Answer from the drawing. Dimensions are ordinates in mm from the lowest x, y and z of the part. Coordinates: 2 decimals unless noted, no trailing zeros. Loops run counter-clockwise (first coordinate to the right, second up) from the corner with the lowest first, then second, coordinate; pieces in that order, holes last. Notation, with made-up numbers: (69, 51.25) - (121, 51.25) arc R18 cw to (121, 65.25) - close; hole circle Ø1 at (73, 75.5). An arc over 180 degrees is marked (long way). Write each question's results on one line, items separated by ' | '. Start each with the question number.
1. A cutting plane is placed at A-A on x = 20. Determine the outline of the cut face in (y, z) (1 decimal), then the cut area to 3 significant figures.
2. A cutting plane is placed at D-D on x = 6. Determine the outline of the cut face in (y, z) (1 decimal), then the cut area to 3 significant figures.
3. This flat-tipped pin is pushed along its axis until it touches: P1, Ø1, axis at x = 23.5, y = 21, coming from the -Z side. Where does it stop, or does it pass through?
4. Determine the mould class of the marked faces 1, 2 and 3 for opening direction Z: released by +Z, released by -Z, zero draft, split by the parting line, or undercut.
5. Find the intervals of material crossed by line 1 along X through (y, z) = (19.75, 25.5); line 2 along Z through (x, y) = (33, 6.5) (1 decimal); line 3 along Z through (x, y) = (21, 18.5) (1 decimal), in increasing order. Write a range as [from, to].
6. A cutting plane is placed at C-C on z = 44. Determine the outline of the cut face in (x, y).
7. A cutting plane is placed at B-B on z = 30. Determine the outline of the cut face in (x, y) (1 decimal), then the cut area to 3 significant figures.
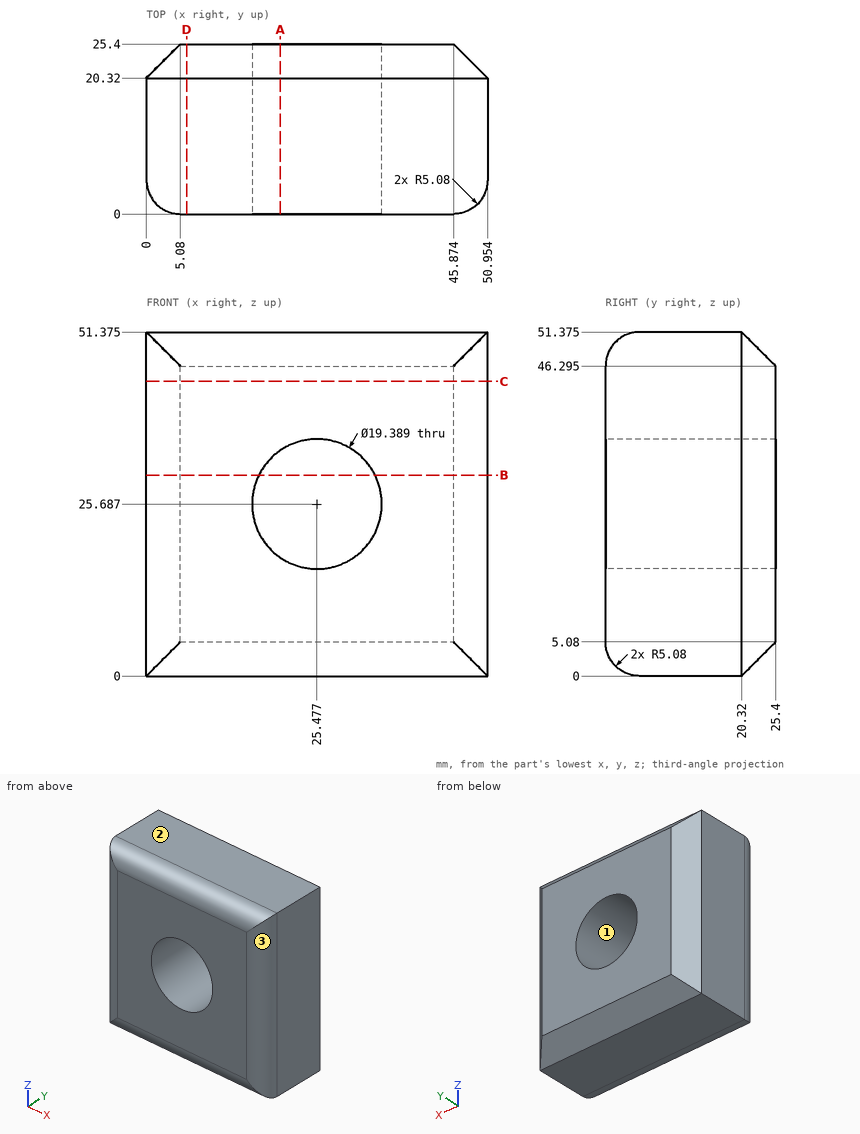
Values:
1) outline: (0, 5.1) arc R5.1 ccw to (5.1, 0) - (20.3, 0) - (25.4, 5.1) - (25.4, 17.7) - (0, 17.7) - close; (0, 33.7) - (25.4, 33.7) - (25.4, 46.3) - (20.3, 51.4) - (5.1, 51.4) arc R5.1 ccw to (0, 46.3) - close | area: 862 mm^2
2) outline: (0, 5.1) arc R5.1 ccw to (5.1, 0) - (20.3, 0) - (25.4, 5.1) - (25.4, 46.3) - (20.3, 51.4) - (5.1, 51.4) arc R5.1 ccw to (0, 46.3) - close | area: 1,270 mm^2
3) P1: z = 0.18
4) face 1: undercut | face 2: released by +Z | face 3: zero draft
5) line 1: [0, 15.78], [35.17, 50.95] | line 2: [0, 19.6], [31.8, 51.4] | line 3: [0, 17.1], [34.3, 51.4]
6) outline: (0, 5.08) arc R5.08 ccw to (5.08, 0) - (45.87, 0) arc R5.08 ccw to (50.95, 5.08) - (50.95, 20.32) - (45.87, 25.4) - (5.08, 25.4) - (0, 20.32) - close
7) outline: (0, 5.1) arc R5.1 ccw to (5.1, 0) - (16.8, 0) - (16.8, 25.4) - (5.1, 25.4) - (0, 20.3) - close; (34.2, 0) - (45.9, 0) arc R5.1 ccw to (51, 5.1) - (51, 20.3) - (45.9, 25.4) - (34.2, 25.4) - close | area: 816 mm^2
